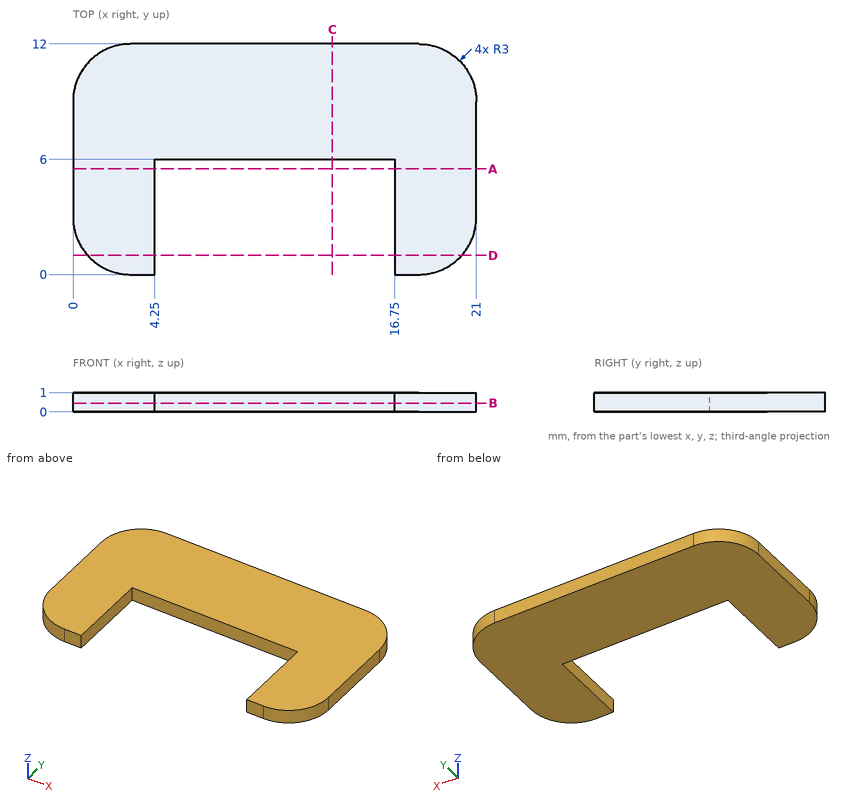
Drawing for the job (mm, zero at the part's lowest x, y, z). Give positions to 0.01 mm unless a question says otherwise; leave off trailing zeros. Order: outer loops, then holes, each group sorted by start corner. A loop starts at its lowest first (then second) coordinate and runs counter-clockwise, first axis right, second up. Notation, with made-up numbers: M 15.5,-3.75 L 46.5,-3.75 A25 cw 46.5,26.25 Z; hole C -34,85.5 d3. An arc over 180 degrees is marked long. Write item = value, one per line. Start each with the question number.
(1) Probe L1, parallel to X at y = 4.5, z = 0.7; L2, parallel to Y at x = 14.5, z = 0.3; L3, parallel to X at y = 11, z = 0.75. List the from-to ranges inside material, lowest first. Write a range as [from, to].
(2) Slice it at B-B on z = 0.45. Write the cut outline in (x, y), plus the area to 3 significant figures.
(3) Slice it at A-A on y = 5.5. Write the cut outline in (x, z), plus the area to 3 significant figures.
(4) Slice it at D-D on y = 1. Write the cut outline in (x, z), plus the area to 3 significant figures.
(5) Slice it at C-C on x = 13.5. Write the cut outline in (y, z).
(6) Pin check, flat tip, straight feed: pin 1 Ø0.5 at (y, z) = (1.5, 0.5) entering from -X. Stop position of the tip, or through.
Responses:
q1.L1 = [0, 4.25], [16.75, 21]
q1.L2 = [6, 12]
q1.L3 = [0.76, 20.24]
q2.outline = M 0,3 A3 ccw 3,0 L 4.25,0 L 4.25,6 L 16.75,6 L 16.75,0 L 18,0 A3 ccw 21,3 L 21,9 A3 ccw 18,12 L 3,12 A3 ccw 0,9 Z
q2.area = 169 mm2
q3.outline = M 0,0 L 4.25,0 L 4.25,1 L 0,1 Z; M 16.75,0 L 21,0 L 21,1 L 16.75,1 Z
q3.area = 8.50 mm2
q4.outline = M 0.76,0 L 4.25,0 L 4.25,1 L 0.76,1 Z; M 16.75,0 L 20.24,0 L 20.24,1 L 16.75,1 Z
q4.area = 6.97 mm2
q5.outline = M 6,0 L 12,0 L 12,1 L 6,1 Z
q6.pin_1 = 0.27
